Answer from the drawing. Dimensions are ordinates in mm from the lowest x, y and z of the part. A direction names the side the tool comes from. Round coordinates to 2 decimals unless told otherwise and drop trailing zeros. Order: outer loops, then holes, each group sorted by start corner. A loop starts at its lowest first (then second) coordinate and runs counter-clockwise, first axis right, second up. Notation, with made-up numbers: (-17, 67.25) -> (22, 67.25) arc R35 ccw to (22, 106.25) -> close; hole circle Ø7 at (32, 10). An arc over 180 degrees is marked (long way). Use a Markdown table: item, result. Add a question column.
1. For the marked faces 1 and 2, determine the directions among +Z, -Z, +X, -X, +Y, -Y from which every point of the face is accessible in a straight line to the end or side of a thin tool.
2. Section B-B, the plane x = 19 is taken. Give the vertices of the cut face in (y, z), then the cut area to 3 significant figures.
3. Section A-A, the plane y = 78 is taken. Give the vertices of the cut face in (x, z), then the cut area to 3 significant figures.
4. Consider L1, parallel to Y at x = 29, z = 2.25; L2, parallel to X at y = 48, z = 0.65; L3, parallel to Y at x = 9, z = 4.45. Determine where each line is inside the solid, lowest interval first. Write a range as [from, to].
5. The mould has two halves that part along Y. Classify the marked faces 3, 4 and 5: +Y half, -Y half, draft (parallel to the pull), parting line (faces both ways), or undercut.
6. Section C-C, the plane y = 62 is taken. Give the vertices of the cut face in (x, z).
7. Section D-D, the plane x = 9 is taken. Give the vertices of the cut face in (y, z).
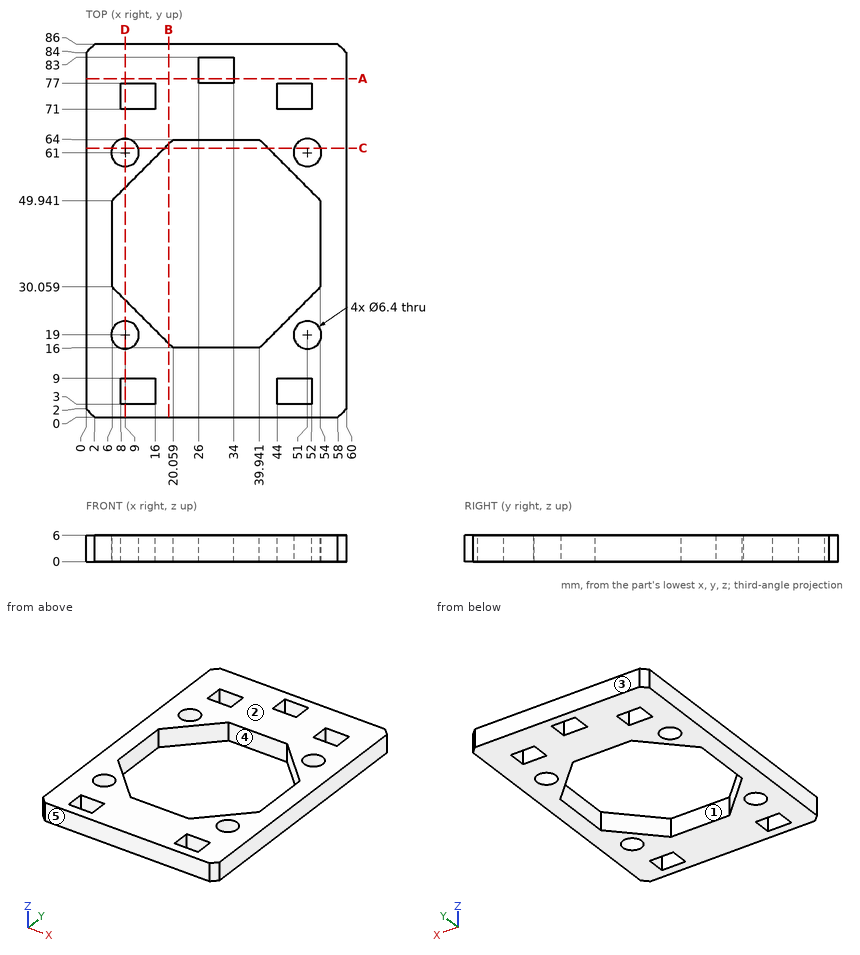
Verdict:
| question | item | result |
|---|---|---|
| 1 | face 1 | +Z, -Z |
| 1 | face 2 | +Z, +X, -X, +Y, -Y |
| 2 | outline | (0, 0) -> (17.06, 0) -> (17.06, 6) -> (0, 6) -> close; (62.94, 0) -> (86, 0) -> (86, 6) -> (62.94, 6) -> close |
| 2 | area | 241 mm2 |
| 3 | outline | (0, 0) -> (26, 0) -> (26, 6) -> (0, 6) -> close; (34, 0) -> (60, 0) -> (60, 6) -> (34, 6) -> close |
| 3 | area | 312 mm2 |
| 4 | L1 | y = [0, 16], [64, 77], [83, 86] |
| 4 | L2 | x = [0, 6], [54, 60] |
| 4 | L3 | y = [0, 3], [9, 15.8], [22.2, 27.06], [52.94, 57.8], [64.2, 71], [77, 86] |
| 5 | face 3 | +Y half |
| 5 | face 4 | undercut |
| 5 | face 5 | -Y half |
| 6 | outline | (0, 0) -> (5.96, 0) -> (5.96, 6) -> (0, 6) -> close; (12.04, 0) -> (18.06, 0) -> (18.06, 6) -> (12.04, 6) -> close; (41.94, 0) -> (47.96, 0) -> (47.96, 6) -> (41.94, 6) -> close; (54.04, 0) -> (60, 0) -> (60, 6) -> (54.04, 6) -> close |
| 7 | outline | (0, 0) -> (3, 0) -> (3, 6) -> (0, 6) -> close; (9, 0) -> (15.8, 0) -> (15.8, 6) -> (9, 6) -> close; (22.2, 0) -> (27.06, 0) -> (27.06, 6) -> (22.2, 6) -> close; (52.94, 0) -> (57.8, 0) -> (57.8, 6) -> (52.94, 6) -> close; (64.2, 0) -> (71, 0) -> (71, 6) -> (64.2, 6) -> close; (77, 0) -> (86, 0) -> (86, 6) -> (77, 6) -> close |
